from build123d import *

# Parameters (mm, degrees)
F0_W     = 120
F0_H     = 60
F0_R     = 15
F1_DEPTH = 5
F2_R     = 5
F3_R     = 15
F4_DEPTH = 5
F5_W     = 20
F5_H     = 60
F6_DEPTH = 2.5


with BuildPart() as f1:
    # F0 (on Top) → F1 (new body)
    with BuildSketch(Plane.XY):
        Rectangle(F0_W, F0_H)
        with Locations((40, 0)):
            Circle(F0_R, mode=Mode.SUBTRACT)
    extrude(amount=F1_DEPTH)

    # F2
    f2_edges = [f1.edges().sort_by_distance(p)[0] for p in [
        (60, 30, 2.5),
        (60, -30, 2.5),
        (-60, -30, 2.5),
        (-60, 30, 2.5),
    ]]
    fillet(f2_edges, radius=F2_R)

    # F3 (on face) → F4 (join)
    with BuildSketch(Plane.XY.offset(5)):
        with Locations((-40, 0)):
            Circle(F3_R)
    extrude(amount=F4_DEPTH)

    # F5 (on face) → F6 (join)
    with BuildSketch(Plane.XY.offset(5)):
        Rectangle(F5_W, F5_H)
    extrude(amount=F6_DEPTH)


solid = f1.part
For this review, take the finished solid that the model builds, in its own axes (mm). A direction names the side the tool comes from. Round coordinates to 2 decimals unless told otherwise and drop trailing zeros. Loops run counter-clockwise (first coordinate to the right, second up) from the corner with the lowest first, then second, coordinate; pieces in that order, holes last. Notation, with made-up numbers: (-5, -1.75) - (19, -1.75) arc R23 cw to (19, 35.25) - close; hole circle Ø6 at (3, -5.5). An arc over 180 degrees is marked (long way). One line per item, written item: value. Start each with the question number.
Item 1: Take a section at C-C (y = 0). Give the boundary of the cut face in (x, z), plus the area to 3 significant figures.
Item 2: Take a section at D-D (x = -40). Give the boundary of the cut face in (y, z).
Item 3: For L1, parallel to Y at x = 40, z = 2.65; L2, parallel to Z at x = -47.5, y = -13.5; L3, parallel to Z at x = -8, y = 17, list the stretches that pass through material, from the lowest coordinate up.
Item 4: The part is to be moulded in two halves that separate along X. For faces 4 (the flat face through (10, 0, 6)), 5 (the flat face through (24, 0, 5)), 6 (the flat face through (-10, 0, 6)), say which applies: +X half, -X half, draft (parallel to the pull), parting line (faces both ways), or undercut.
Item 5: Take a section at A-A (x = 40). Give the boundary of the cut face in (y, z), plus the area to 3 significant figures.
Item 6: Take a section at B-B (z = 6.25). Give the boundary of the cut face in (x, y), plus the area to 3 significant figures.
Item 7: Clearance check with flat-ended pins moving along their axes: pin 1 Ø18 at (x, y) = (40, 0) entering from -Z; pin 2 Ø22 at (x, y) = (-2.5, 15) entering from +Z; pin 3 Ø0.8 at (y, z) = (2.5, 6.5) entering from -X; pin 4 Ø15 at (x, y) = (47, -6) entering from +Z. State where each tip first meets the part, or that it passes through.
Item 8: For faces 1 (the cylindrical face through (-59, 28, 3)), 2 (the flat face through (0, 0, 7.5)), 3 (the cylindrical face through (-54.985, 0.66, 7.465)), list the 3-axis set-ups (+Z, -Z, +X, -X, +Y, -Y) from which the entire face can be reached by the end or side of a thin tool; tool diameter is ignored.
Answer below:
1. outline: (-60, 0) - (25, 0) - (25, 5) - (10, 5) - (10, 7.5) - (-10, 7.5) - (-10, 5) - (-25, 5) - (-25, 10) - (-55, 10) - (-55, 5) - (-60, 5) - close; (55, 0) - (60, 0) - (60, 5) - (55, 5) - close
1. area: 650 mm2
2. outline: (-30, 0) - (30, 0) - (30, 5) - (15, 5) - (15, 10) - (-15, 10) - (-15, 5) - (-30, 5) - close
3. L1: y = -30 to -15, 15 to 30
3. L2: z = 0 to 5
3. L3: z = 0 to 7.5
4. face 4: +X half
4. face 5: draft
4. face 6: undercut
5. outline: (-30, 0) - (-15, 0) - (-15, 5) - (-30, 5) - close; (15, 0) - (30, 0) - (30, 5) - (15, 5) - close
5. area: 150 mm2
6. outline: circle Ø30 at (-40, 0); (-10, -30) - (10, -30) - (10, 30) - (-10, 30) - close
6. area: 1,910 mm2
7. pin 1: passes through
7. pin 2: stops at z = 7.5
7. pin 3: stops at x = -54.85
7. pin 4: stops at z = 5
8. face 1: +Z, -Z, -X, +Y
8. face 2: +Z, +X, +Y, -Y
8. face 3: +Z
